Build history of the part. All positions in model axes, mm. A direction names the side the tool comes from. Round coordinates to 2 decimals unless told otherwise and drop trailing zeros. Order: outer loops, then holes, each group sorted by start corner. A loop starts at its lowest first (then second) coordinate and runs counter-clockwise, first axis right, second up. Notation, with made-up numbers: (36.25, -33) -> (40.25, -33) arc R27 ccw to (40.25, -10) -> close; hole circle Ø7 at (-2.75, 88.5). An arc over 180 degrees is marked (long way). Answer as a JSON object with one key per item and string values.
from build123d import *

# Parameters (mm, degrees)
SKETCH1_W               = 130
SKETCH1_H               = 26.5
BOSS_EXTRUDE2_DEPTH     = 15
CUT_EXTRUDE1_DEPTH      = 132.531602666
CUT_EXTRUDE1_DEPTH_BACK = 132.531602666
SKETCH4_W               = 5
SKETCH4_H               = 7
BOSS_EXTRUDE3_DEPTH     = 8
BOSS_EXTRUDE4_DEPTH     = 3.5
SKETCH5_3_W             = 1
SKETCH5_3_H             = 8
CUT_EXTRUDE2_DEPTH      = 3.5


with BuildPart() as part:
    # Sketch1 → Boss-Extrude2 (new body)
    with BuildSketch(Plane(origin=(0, 0, 0), x_dir=(1, 0, 0), z_dir=(0, 1, 0))):
        Rectangle(SKETCH1_W, SKETCH1_H)
    extrude(amount=BOSS_EXTRUDE2_DEPTH)

    # Sketch2 → Cut-Extrude1 (cut, two sides: drawn at the far end of the back side and taken through both)
    with BuildSketch(Plane.ZY.offset(65).offset(-CUT_EXTRUDE1_DEPTH_BACK)):
        with BuildLine():
            Line((-4.434381462, 1.80539147), (13.25, 7.838944467))
            Line((13.25, 7.838944467), (13.25, 15))
            Line((13.25, 15), (-9.725995121, 15))
            Line((-9.725995121, 15), (-9.725995121, 5.591119162))
            ThreePointArc((-9.725995121, 5.591119162), (-8.053391237, 2.337931907), (-4.434381462, 1.80539147))
        make_face()
    extrude(amount=CUT_EXTRUDE1_DEPTH + CUT_EXTRUDE1_DEPTH_BACK, mode=Mode.SUBTRACT)

    # Sketch4 → Boss-Extrude3 (add)
    with BuildSketch(Plane.XZ):
        with Locations((-42.5, -4.75)):
            Rectangle(SKETCH4_W, SKETCH4_H)
        with Locations((42.5, -4.75)):
            Rectangle(SKETCH4_W, SKETCH4_H)
    extrude(amount=BOSS_EXTRUDE3_DEPTH)

    # Sketch5 → Boss-Extrude4 (add, symmetric)
    with BuildSketch(Plane.XY.offset(-4.75)):
        Polygon((-45, -8), (-45, -5), (-46, -5), align=None)
        Polygon((-40, -5), (-40, -8), (-39, -5), align=None)
        Polygon((46, -5), (45, -5), (45, -8), align=None)
        Polygon((40, -8), (40, -5), (39, -5), align=None)
    extrude(amount=BOSS_EXTRUDE4_DEPTH, both=True)

    # Sketch5<3> → Cut-Extrude2 (cut, symmetric)
    with BuildSketch(Plane.XY.offset(-4.75)):
        with Locations((-42.5, -4)):
            Rectangle(SKETCH5_3_W, SKETCH5_3_H)
        with Locations((42.5, -4)):
            Rectangle(SKETCH5_3_W, SKETCH5_3_H)
    extrude(amount=CUT_EXTRUDE2_DEPTH, both=True, mode=Mode.SUBTRACT)


solid = part.part
1) Probe L1, parallel to X at y = -3.5, z = -8; L2, parallel to Z at x = 57, y = 12.25; L3, parallel to Y at x = -13, z = -6. List the from-to ranges inside material, lowest first. Write a range as from..to.
Checked values:
{"L1": "x = -45..-43, -42..-40, 40..42, 43..45", "L2": "z = -13.25..-9.73", "L3": "y = 0..1.6"}
2) Cut at A-A, the plane y = 3.5. Give the cut face in (x, z).
Checked values:
{"outline": "(-65, -13.25) -> (65, -13.25) -> (65, -9.14) -> (-65, -9.14) -> close; (-65, 0.53) -> (65, 0.53) -> (65, 13.25) -> (-65, 13.25) -> close"}
3) Cut at B-B, the plane x = -30.5. Give the cut face in (y, z).
Checked values:
{"outline": "(0, -13.25) -> (15, -13.25) -> (15, -9.73) -> (5.59, -9.73) arc R4 cw to (1.81, -4.43) -> (7.84, 13.25) -> (0, 13.25) -> close"}
4) Cut at D-D, the plane y = 9.5. Give the cut face in (x, z).
Checked values:
{"outline": "(-65, -13.25) -> (65, -13.25) -> (65, -9.73) -> (-65, -9.73) -> close"}
5) Which spindle directions (+Z, -Z, +X, -X, +Y, -Y) get a long thin tool onto all of the face, cutting with end or side? Do faces 1 (the face through (1, 10, -9.726)), 2 (the face through (-42, -4, -5)), 3 (the face through (44, -4, -8.25)), 4 (the face through (-1, 4, 13.25)), 5 (the face through (41, -4, -1.25)). Say none if no direction does.
Checked values:
{"face 1": "+X, -X, +Y", "face 2": "+Z, -Z, -Y", "face 3": "-Z, +X, -X, -Y", "face 4": "+Z, +X, -X, +Y, -Y", "face 5": "+Z, +X, -X, -Y"}
6) Cut at C-C, the plane z = -6.25. Give the cut face in (x, y), plus the area to 3 significant figures.
Checked values:
{"outline": "(-65, 0) -> (-45, 0) -> (-45, -5) -> (-46, -5) -> (-45, -8) -> (-43, -8) -> (-43, 0) -> (-42, 0) -> (-42, -8) -> (-40, -8) -> (-39, -5) -> (-40, -5) -> (-40, 0) -> (40, 0) -> (40, -5) -> (39, -5) -> (40, -8) -> (42, -8) -> (42, 0) -> (43, 0) -> (43, -8) -> (45, -8) -> (46, -5) -> (45, -5) -> (45, 0) -> (65, 0) -> (65, 1.63) -> (-65, 1.63) -> close", "area": "281 mm²"}
7) Pull direction X, two halves, no side cores. Call faces 6 (the face through (-39.5, -6.5, -4.8)), 7 (the face through (-41, -4, -8.25)), 8 (the face through (-45.5, -6.5, -4.8)): pulls with the +X half, pulls with the -X half, needs draft (parallel to the pull), parting line crosses it, or undercut.
Checked values:
{"face 6": "undercut", "face 7": "needs draft", "face 8": "pulls with the -X half"}
8) Flat gauge pins, fed straight in: pin 1 Ø1 at (y, z) = (6.5, 3.5) entering from -X; pin 2 Ø2 at (x, z) = (46.5, 0) entering from -Y; pin 3 Ø7.5 at (y, z) = (-5.5, -6) entering from -X; pin 4 Ø1.1 at (x, z) = (-39.5, -4.5) entering from +Y. Where does each tip first touch, or does it go through?
Checked values:
{"pin 1": "passes through", "pin 2": "stops at y = 0", "pin 3": "stops at x = -46", "pin 4": "stops at y = 1.97"}
